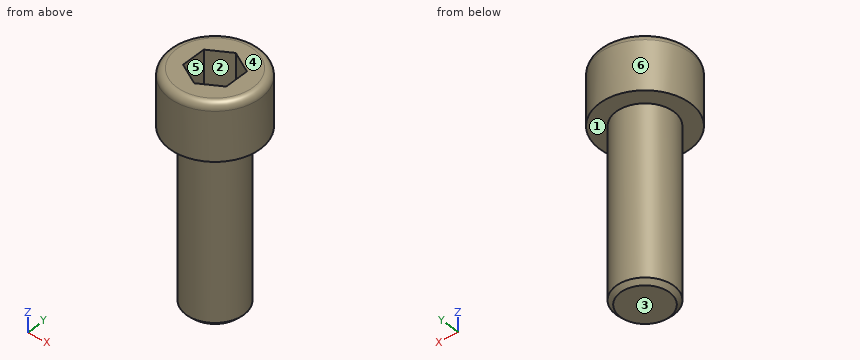
```python
from build123d import *

# Parameters (mm, degrees)
CUT_EXTRUDE_1_DEPTH = 2.5
FILLET_1_R          = 0.5
CHAMFER_1_SIZE      = 0.3


with BuildPart() as part:
    # 草图1 → 旋转1 (revolve)
    with BuildSketch(Plane(origin=(0, 0, 0), x_dir=(0, 0, -1), z_dir=(1, 0, 0))):
        Polygon((-7.95, 0), (-7.95, 3.15), (-4.05, 3.15), (-4.05, 2), (7.95, 2), (7.95, 0), align=None)
    revolve(axis=Axis((0, 0, -7.95), (0, 0, 1)))

    # 草图2 → 切除-拉伸1 (cut)
    with BuildSketch(Plane.XY.offset(7.95)):
        Polygon((0, 1.732050808), (-1.5, 0.866025404), (-1.5, -0.866025404), (0, -1.732050808), (1.5, -0.866025404), (1.5, 0.866025404), align=None)
    extrude(amount=-CUT_EXTRUDE_1_DEPTH, mode=Mode.SUBTRACT)

    # 圆角1
    fillet_1_edges = [part.edges().sort_by_distance(p)[0] for p in [
        (0, -3.15, 7.95),
    ]]
    fillet(fillet_1_edges, radius=FILLET_1_R)

    # 倒角1
    chamfer_1_edges = [part.edges().sort_by_distance(p)[0] for p in [
        (0, -2, -7.95),
    ]]
    chamfer(chamfer_1_edges, length=CHAMFER_1_SIZE)


solid = part.part
```
Build history of the part. All positions in model axes, mm. Face numbers are marked on the shaded views. A direction names the side the tool comes from. Round coordinates to 2 decimals unless told otherwise and drop trailing zeros. Loops run counter-clockwise (first coordinate to the right, second up) from the corner with the lowest first, then second, coordinate; pieces in that order, holes last.
Item 1: Saw through at B-B (y = 0). List the corners of the cut face in (x, z).
Item 2: Which spindle directions (+Z, -Z, +X, -X, +Y, -Y) get a long thin tool onto all of the face, cutting with end or side? Do the marked faces 1, 2 and 3. Say none if no direction does.
Item 3: Saw through at C-C (z = -6). List the corners of the cut face in (x, y), then the cut area to 3 significant figures.
Item 4: Drill centre lines: line 1 along Y through (x, z) = (1, -1); line 2 along Z through (x, y) = (0.75, -1); line 3 along Y through (x, z) = (0, -6.25). Where is each one in solid material? Low to high.
Item 5: Two-plate mould, pull along X, no slides. Class the marked faces 4, 5 and 6: released by +X, released by -X, zero draft, split by the parting line, or undercut.
Item 6: Pin check, flat tip, straight feed: P1, Ø2, axis at x = -2, z = -5.5, coming from the -Y side. Stop position of the tip, or through.
Item 7: Saw through at A-A (z = 5.75). List the corners of the cut face in (x, y).
Worked answers:
1. outline: (-3.15, 4.05) - (-2, 4.05) - (-2, -7.65) - (-1.7, -7.95) - (1.7, -7.95) - (2, -7.65) - (2, 4.05) - (3.15, 4.05) - (3.15, 7.45) arc R0.5 ccw to (2.65, 7.95) - (1.5, 7.95) - (1.5, 5.45) - (-1.5, 5.45) - (-1.5, 7.95) - (-2.65, 7.95) arc R0.5 ccw to (-3.15, 7.45) - close
2. face 1: -Z
2. face 2: +Z
2. face 3: -Z, +X, -X, +Y, -Y
3. outline: circle Ø4 at (0, 0)
3. area: 12.6 mm2
4. line 1: y = -1.73 to 1.73
4. line 2: z = -7.95 to 5.45
4. line 3: y = -2 to 2
5. face 4: zero draft
5. face 5: undercut
5. face 6: split by the parting line
6. P1: stops at y = -1.73
7. outline: circle Ø6.3 at (0, 0); hole (-1.5, -0.87) - (0, -1.73) - (1.5, -0.87) - (1.5, 0.87) - (0, 1.73) - (-1.5, 0.87) - close
